Check sheet for the modelled part. Datum: model origin and axes. Units: mm. A direction names the side the tool comes from. Round coordinates to 2 decimals unless told otherwise and drop trailing zeros. Order: outer loops, then holes, each group sorted by start corner. A loop starts at its lowest first (then second) coordinate and runs counter-clockwise, first axis right, second up. Notation, with made-up numbers: (-11.5, -26) -> (16.5, -26) arc R5 ccw to (16.5, -22) -> close; hole circle Ø1 at (14, -0.75). An arc over 180 degrees is marked (long way). Answer in a Markdown table with one row per item.
```python
from build123d import *

# Parameters (mm, degrees)
F0_W     = 2000
F0_H     = 265
F1_DEPTH = 38
F2_R     = 5
F3_W     = 44.824789
F3_H     = 380.666598
F3_W_2   = 70.77609
F3_H_2   = 364.249266
F4_DEPTH = 19
F5_W     = 38
F5_H     = 342.808559
F5_H_2   = 434.554458
F6_DEPTH = 19


with BuildPart() as f1:
    # F0 (on Top) → F1 (new body)
    with BuildSketch(Plane.XY):
        with Locations((2.617415, -379.390822)):
            Rectangle(F0_W, F0_H)
    extrude(amount=F1_DEPTH)

    # F2
    f2_edges = [f1.edges().sort_by_distance(p)[0] for p in [
        (2.617415, -246.890822, 38),
        (-997.382585, -379.390822, 38),
        (2.617415, -511.890822, 38),
        (1002.617415, -379.390822, 38),
        (2.617415, -246.890822, 0),
        (-997.382585, -379.390822, 0),
        (2.617415, -511.890822, 0),
        (1002.617415, -379.390822, 0),
    ]]
    fillet(f2_edges, radius=F2_R)

    # F3 (on face) → F4 (cut)
    with BuildSketch(Plane(origin=(0, 0, 0), x_dir=(1, 0, 0), z_dir=(0, 0, -1))):
        with Locations((-981.794979, 384.322472)):
            Rectangle(F3_W, F3_H)
        with Locations((1000.00546, 386.361368)):
            Rectangle(F3_W_2, F3_H_2)
    extrude(amount=-F4_DEPTH, mode=Mode.SUBTRACT)

    # F5 (on face) → F6 (cut)
    with BuildSketch(Plane(origin=(0, 0, 0), x_dir=(1, 0, 0), z_dir=(0, 0, -1))):
        with Locations((-325.382585, 353.463552)):
            Rectangle(F5_W, F5_H)
        with Locations((330.617415, 355.673134)):
            Rectangle(F5_W, F5_H_2)
    extrude(amount=-F6_DEPTH, mode=Mode.SUBTRACT)


solid = f1.part
```
(1) Depth check by flat-ended pin: pin 1 Ø4 at (y, z) = (-429.5, 4.5) entering from +X; pin 2 Ø11.5 at (x, y) = (-316.5, -410) entering from -Z; pin 3 Ø1.5 at (y, z) = (-303.5, 5) entering from -X. Enter the tip coordinate at first touch or a pass-through.
Solutions:
| item | result |
|---|---|
| pin 1 | x = 964.62 |
| pin 2 | z = 19 |
| pin 3 | x = -959.38 |
(2) Tool access check on faces 1 (the flat face through (-979, -381, 19)), 2 (the flat face through (983, -381, 19)), 3 (the flat face through (-11, -378, 38)). Record the directions out of +Z, -Z, +X, -X, +Y, -Y that give a thin tool (end or side, any length) a straight path to the whole face; none if there is none.
Solutions:
| item | result |
|---|---|
| face 1 | -Z, -X, +Y, -Y |
| face 2 | -Z, +X, +Y, -Y |
| face 3 | +Z, +X, -X, +Y, -Y |
(3) Scan lines: probe 1 along X at (y, z) = (-394.5, 17); probe 2 along Y at (x, z) = (-43.5, 34.5); probe 3 along Z at (x, y) = (-331, -432). Record each from-to range of solid material in increasing order. Write a range as from..to.
Solutions:
| item | result |
|---|---|
| probe 1 | -959.38..-344.38, -306.38..311.62, 349.62..964.62 |
| probe 2 | -511.66..-247.12 |
| probe 3 | 19..38 |
(4) Section check A-A on z = 12.5. Record the boundary of the cut face in (x, y), plus the area to 3 significant figures.
Solutions:
| item | result |
|---|---|
| outline | (-959.38, -511.89) -> (-344.38, -511.89) -> (-344.38, -246.89) -> (-959.38, -246.89) -> close; (-306.38, -511.89) -> (311.62, -511.89) -> (311.62, -246.89) -> (-306.38, -246.89) -> close; (349.62, -511.89) -> (964.62, -511.89) -> (964.62, -246.89) -> (349.62, -246.89) -> close |
| area | 490,000 mm^2 |
(5) Section check B-B on y = -427.5. Record the boundary of the cut face in (x, z).
Solutions:
| item | result |
|---|---|
| outline | (-997.38, 19) -> (-959.38, 19) -> (-959.38, 0) -> (-344.38, 0) -> (-344.38, 19) -> (-306.38, 19) -> (-306.38, 0) -> (311.62, 0) -> (311.62, 19) -> (349.62, 19) -> (349.62, 0) -> (964.62, 0) -> (964.62, 19) -> (1002.62, 19) -> (1002.62, 33) arc R5 ccw to (997.62, 38) -> (-992.38, 38) arc R5 ccw to (-997.38, 33) -> close |
(6) Draft check along X on faces 4 (the flat face through (330, -381, 19)), 5 (the flat face through (-656, -378, 0)), 6 (the flat face through (-326, -381, 19)). Enter one of: pulls with the +X half, pulls with the -X half, needs draft (parallel to the pull), parting line crosses it, or undercut.
Solutions:
| item | result |
|---|---|
| face 4 | undercut |
| face 5 | needs draft |
| face 6 | undercut |
